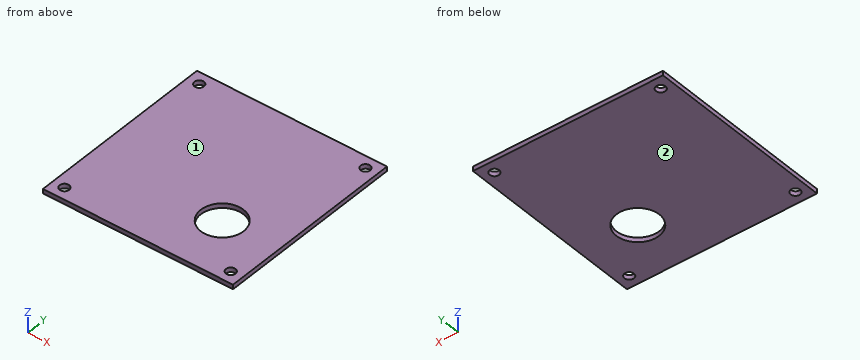
Autodesk Inventor part; units mm, degrees
ref_plane "YZ Plane" through (0, 0, 0) normal (1, 0, 0) x (0, 1, 0)
ref_plane "XZ Plane" through (0, 0, 0) normal (0, 1, 0) x (-1, 0, 0)
ref_plane "XY Plane" through (0, 0, 0) normal (0, 0, 1) x (1, 0, 0)
sketch "Sketch1" plane through (0, 0, 0) normal (0, 0, 1) x (1, 0, 0)
  line L0 (0, 0) -> (127, 0)
  line L1 (127, 0) -> (127, 127)
  line L2 (127, 127) -> (0, 127)
  line L3 (0, 127) -> (0, 0)
  dimension "d0" = 127
extrude "Plate1" add sketch "Sketch1" along normal blind 3.048
sketch "gbmh_sketch" plane through (0, 0, 3.048) normal (0, 0, 1) x (1, 0, 0)
  line L0 (7.9248, 119.0752) -> (119.0752, 119.0752) construction
  line L1 (127, 127) -> (0, 127) construction
  line L2 (119.0752, 119.0752) -> (119.0752, 7.9248) construction
  line L3 (119.0752, 7.9248) -> (7.9248, 7.9248) construction
  line L4 (7.9248, 7.9248) -> (7.9248, 119.0752) construction
  line L5 (7.9248, 119.0752) -> (7.9248, 127) construction
  line L6 (7.9248, 119.0752) -> (0, 119.0752) construction
  line L7 (0, 127) -> (0, 0) construction
  line L8 (119.0752, 7.9248) -> (127, 7.9248) construction
  line L9 (127, 0) -> (127, 127) construction
  line L10 (119.0752, 7.9248) -> (119.0752, 0) construction
  dimension "d2" = 111.1504
  dimension "d3" = 111.1504
  dimension "d4" = 111.1504
  dimension "d5" = 111.1504
hole "gbmh" at (7.9248, 119.0752, 3.048) at (7.9248, 7.9248, 3.048) at (119.0752, 7.9248, 3.048) at (119.0752, 119.0752, 3.048) direction (0, 0, -1) diameter 6.35 depth 3.048 tip angle 118
sketch "bearing_hole_sketch" plane through (0, 0, 3.048) normal (0, 0, 1) x (1, 0, 0)
  line L0 (127, 0) -> (0, 0)
  line L1 (127, 127) -> (127, 0)
  point P0 (88.9, 38.1)
  dimension "d13" = 38.1
  dimension "d14" = 38.1
hole "ss_bearing_hole" at (88.9, 38.1, 3.048) direction (0, 0, -1) diameter 28.575 depth 3.048 tip angle 118
equation "\"d6\" = gb_mh_diameter"
equation "\"d11\" = Thickness"
equation "\"d15\" = gb_bearing_diameter"
equation "\"d20\" = Thickness"
equation "\"BendRadius\" = Thickness"
equation "\"BendReliefWidth\" = Thickness"
equation "\"BendReliefDepth\" = 0.5 * Thickness"
equation "\"CornerReliefSize\" = 4 * Thickness"
equation "\"MinimumRemnant\" = 2 * Thickness"
equation "\"TransitionRadius\" = BendRadius"
equation "\"JacobiRadiusSize\" = BendRadius"
equation "\"GapSize\" = Thickness"
equation "\"d1\" = BendRadius"
equation "\"gb_mh_seperation\" = 111.1504"
equation "\"gb_mh_diameter\" = 6.35"
equation "\"gb_axle_from_edge\" = 38.1"
equation "\"gb_width\" = 127"
equation "\"gb_bearing_diameter\" = 28.575"
equation "\"gb_to_bottom_of_side_assembly\" = 4.7752"
equation "\"gb_mh_seperation_alt\" = 111.125"
equation "\"gb_axle_from_edge_alt\" = 43.1546"
properties part number "gearboxbearingplate(gbpb)" material "Aluminum 6061"
Geometry check sheet. Reference: the model listing, model coordinates, mm. Face numbers are marked on the shaded views. Coordinates: 2 decimals unless noted, no trailing zeros. Write each loop counter-clockwise with the first axis right and the second up, starting at its lowest first coordinate (ties: lowest second). Pieces come first, ordered by that corner, then holes. Notation, with made-up numbers: M -25,46 L -6,46 A24 ccw -6,73 Z; hole C -8.75,56 d7. An arc over 180 degrees is marked long. Use one line per item in the form item = value. Start each with the question number.
1) Thickness scan on probe 1 along X at (y, z) = (38.1, 1.8); probe 2 along X at (y, z) = (122, 2.2); probe 3 along Y at (x, z) = (88.9, 1.25). Record the ranges inside material, lowest first. Write a range as from..to.
2) Section check A-A on y = 38.1. Enter the section's corners in (x, z).
3) Section check C-C on z = 2.5. State how many separate pieces and enclosed holes the cut face has, and give its area (3 significant figures).
4) Release check for a two-part mould opening along Z. For the marked faces 1 and 2 record: pulls with the +Z half, pulls with the -Z half, needs draft (parallel to the pull), parting line crosses it, or undercut.
5) Section check B-B on x = 88.9. Enter the section's corners in (y, z).
Responses:
q1.probe_1 = 0..74.61, 103.19..127
q1.probe_2 = 0..6.69, 9.16..117.84, 120.31..127
q1.probe_3 = 0..23.81, 52.39..127
q2.outline = M 0,0 L 74.61,0 L 74.61,3.05 L 0,3.05 Z; M 103.19,0 L 127,0 L 127,3.05 L 103.19,3.05 Z
q3.separate_pieces = 1
q3.enclosed_holes = 5
q3.area = 15,400 mm2
q4.face_1 = pulls with the +Z half
q4.face_2 = pulls with the -Z half
q5.outline = M 0,0 L 23.81,0 L 23.81,3.05 L 0,3.05 Z; M 52.39,0 L 127,0 L 127,3.05 L 52.39,3.05 Z
